```python
from build123d import *

# Parameters (mm, degrees)
SKETCH2_R               = 3.999992
BOSS_EXTRUDE1_DEPTH     = 16.301974
CUT_EXTRUDE1_REACH      = 30.308
CUT_EXTRUDE1_END_RADIUS = 3.999992
SKETCH3_R               = 3.175


with BuildPart() as part:
    # Sketch2 → Boss-Extrude1 (new body)
    with BuildSketch(Plane.XY):
        with BuildLine():
            Line((-10.349992, 0), (-10.349992, 10.349992))
            Line((-10.349992, 10.349992), (0, 10.349992))
            Line((0, 10.349992), (10.349992, 10.349992))
            Line((10.349992, 10.349992), (10.349992, 0))
            ThreePointArc((10.349992, 0), (0, -10.349992), (-10.349992, 0))
        make_face()
        Circle(SKETCH2_R, mode=Mode.SUBTRACT)
    extrude(amount=BOSS_EXTRUDE1_DEPTH)

    # Cut-Extrude1: up to this cylinder (the profile starts outside it)
    cut_extrude1_end = Plane(origin=(0, 0, 8.150987), z_dir=(0, 0, -1)) * Cylinder(CUT_EXTRUDE1_END_RADIUS, 69.615984, mode=Mode.PRIVATE)
    # Sketch3 → Cut-Extrude1 (cut, up to the surface)
    with BuildSketch(Plane(origin=(0, 10.349992, 0), x_dir=(1, 0, 0), z_dir=(0, 1, 0)), mode=Mode.PRIVATE) as cut_extrude1_sk1:
        with Locations(Location((0, -8.150987, 0), (0, 0, 270))):
            Circle(SKETCH3_R)
    cut_extrude1_tool1 = extrude(cut_extrude1_sk1.sketch, amount=-CUT_EXTRUDE1_REACH, mode=Mode.PRIVATE) - cut_extrude1_end
    add(cut_extrude1_tool1.solids().sort_by_distance((0, 10.349992, 8.150987))[0], mode=Mode.SUBTRACT)


solid = part.part
```
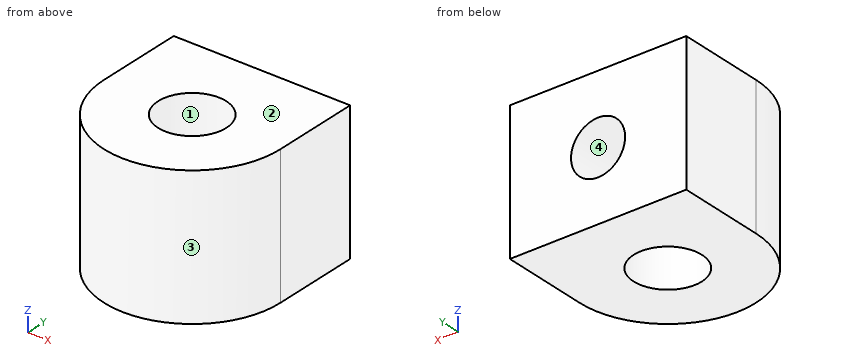
Verification items for the finished model (mm, model axes). Face numbers are marked on the shaded views. Round coordinates to 2 decimals unless told otherwise and drop trailing zeros. Order: outer loops, then holes, each group sorted by start corner. A loop starts at its lowest first (then second) coordinate and runs counter-clockwise, first axis right, second up.
1) Draft check along X on the marked faces 1, 2, 3 and 4. Enter one of: +X half, -X half, draft (parallel to the pull), parting line (faces both ways), or undercut.
Geometry says:
face 1: undercut
face 2: draft
face 3: parting line
face 4: undercut
2) Material ranges on line 1 (Z direction, x = 0, y = 5.25); line 2 (Y direction, x = 2.5, z = 2.75); line 3 (Y direction, x = 0, z = 9), recorded low to high.
Geometry says:
line 1: z = 0 to 4.98, 11.33 to 16.3
line 2: y = -10.04 to -3.12, 3.12 to 10.35
line 3: y = -10.35 to -4
3) Cross-section at C-C, the plane y = -2. Record the cut outline in (x, z).
Geometry says:
outline: (-10.15, 0) - (-3.46, 0) - (-3.46, 16.3) - (-10.15, 16.3) - close; (3.46, 0) - (10.15, 0) - (10.15, 16.3) - (3.46, 16.3) - close
4) Cross-section at A-A, the plane x = 0. Record the cut outline in (y, z), plus the area to 3 significant figures.
Geometry says:
outline: (-10.35, 0) - (-4, 0) - (-4, 16.3) - (-10.35, 16.3) - close; (4, 0) - (10.35, 0) - (10.35, 4.98) - (4, 4.98) - close; (4, 11.33) - (10.35, 11.33) - (10.35, 16.3) - (4, 16.3) - close
area: 167 mm2
5) Depth check by flat-ended pin: pin 1 (4 mm diameter, centred on y = -5.5, z = 7.5, fed in from +X). Enter the tip coordinate at first touch or a pass-through.
Geometry says:
pin 1: stops at x = 9.74
6) Cross-section at B-B, the plane z = 13.25. Record the cut outline in (x, y).
Geometry says:
outline: (-10.35, 0) arc R10.35 ccw to (10.35, 0) - (10.35, 10.35) - (-10.35, 10.35) - close; hole circle Ø8 at (0, 0)
7) Cross-section at D-D, the plane z = 7.75. Record the cut outline in (x, y).
Geometry says:
outline: (-10.35, 0) arc R10.35 ccw to (10.35, 0) - (10.35, 10.35) - (3.15, 10.35) - (3.15, 2.47) arc R4 cw (long way) to (-3.15, 2.47) - (-3.15, 10.35) - (-10.35, 10.35) - close
